```python
from build123d import *

# Parameters (mm, degrees)
CUT_EXTRUDE_1_DEPTH      = 192.109261942
CUT_EXTRUDE_1_DEPTH_BACK = 192.109261942
SKETCH_2_W               = 30
SKETCH_2_H               = 7.5
CHAMFER_1_SIZE           = 1.5
M8X1_01_D                = 7
M8X1_01_DEPTH            = 20
M8X1_01_CSINK_D          = 10
M8X1_01_CSINK_ANGLE      = 90
M8X1_01_TIP              = 2.103012167


with BuildPart() as part:
    # Эскиз1 → Повернуть1 (revolve)
    with BuildSketch(Plane.XY, mode=Mode.PRIVATE) as revolve_1_sk:
        Polygon((-186.5, 0), (-186.5, 25), (-82.5, 25), (-82.5, 29.5), (82.5, 29.5), (82.5, 25), (145.5, 25), (145.5, 0), align=None)
    revolve(revolve_1_sk.sketch.rotate(Axis((0, 0, 0), (-1, 0, 0)), 90), axis=Axis((0, 0, 0), (-1, 0, 0)))

    # Эскиз2 → Вырез-Вытянуть1 (cut, two sides: drawn at the far end of the back side and taken through both)
    with BuildSketch(Plane(origin=(0, 0, 0), x_dir=(1, 0, 0), z_dir=(0, 1, 0)).offset(-CUT_EXTRUDE_1_DEPTH_BACK)):
        with Locations((-171.5, 21.25)):
            Rectangle(SKETCH_2_W, SKETCH_2_H)
        with Locations((-171.5, -21.25)):
            Rectangle(SKETCH_2_W, SKETCH_2_H)
        with Locations((130.5, 21.25)):
            Rectangle(SKETCH_2_W, SKETCH_2_H)
        with Locations((130.5, -21.25)):
            Rectangle(SKETCH_2_W, SKETCH_2_H)
    extrude(amount=CUT_EXTRUDE_1_DEPTH + CUT_EXTRUDE_1_DEPTH_BACK, mode=Mode.SUBTRACT)

    # Фаска1
    chamfer_1_edges = [part.edges().sort_by_distance(p)[0] for p in [
        (145.5, 25, 0),
        (145.5, -25, 0),
        (-186.5, 25, 0),
        (-186.5, -25, 0),
        (82.5, 0, 29.5),
        (-82.5, 0, 29.5),
    ]]
    chamfer(chamfer_1_edges, length=CHAMFER_1_SIZE)

    # Отверстие обработанное метчиком M8x1.01
    with Locations(Plane(origin=(-172.5, 25, 0), x_dir=(0, 0, 1), z_dir=(0, 1, 0))):
        with Locations((0, 0), (0, 305)):
            CounterSinkHole(M8X1_01_D / 2, M8X1_01_CSINK_D / 2, depth=M8X1_01_DEPTH, counter_sink_angle=M8X1_01_CSINK_ANGLE)
            with Locations((0, 0, -(M8X1_01_DEPTH + M8X1_01_TIP / 2))):  # 118° drill point
                Cone(0, M8X1_01_D / 2, M8X1_01_TIP, mode=Mode.SUBTRACT)


solid = part.part
```
The model under review builds one solid part; all positions refer to its coordinate system, in mm. A direction names the side the tool comes from. Give positions to 0.01 mm unless a question says otherwise; leave off trailing zeros. Loops run counter-clockwise (first coordinate to the right, second up) from the corner with the lowest first, then second, coordinate; pieces in that order, holes last. Notation, with made-up numbers: (-5, 23.25) -> (-1, 23.25) arc R23 cw to (-1, 45.25) -> close; hole circle Ø1 at (5, -31). An arc over 180 degrees is marked (long way). Use CSV: the item, a comma, the result in double quotes.
1. To check wall thickness, follow probe 1 along X at (y, z) = (9, 0); probe 2 along Z at (x, y) = (132.5, 15); probe 3 along Y at (x, z) = (-78, -1). State the ranges of each line that lie inside material, in increasing order. Write a range as from..to.
Result:
probe 1,"x = -186.5..-176, -169..129, 136..145.5"
probe 2,"z = -17.5..-3.5, 3.5..17.5"
probe 3,"y = -29.48..29.48"
2. Consider section C-C, the plane x = -59.5. Write out the cut boundary in (y, z), then the cut area to 3 significant figures.
Result:
outline,"circle Ø59 at (0, 0)"
area,"2,730 mm²"
3. For P1, Ø2, axis at x = -96.5, y = -10.5, coming from the +Z side; P2, Ø2, axis at y = -6.5, z = 20.5, coming from the -X side; P3, Ø9, axis at x = 135, y = -5, coming from the -Z side, all flat-tipped, find the tip position at first contact; note any pin that passes through.
Result:
P1,"stops at z = 23.12"
P2,"stops at x = -156.5"
P3,"stops at z = -17.5"
4. Consider section B-B, the plane x = 124. Write out the cut boundary in (y, z), then the cut area to 3 significant figures.
Result:
outline,"(-17.85, -17.5) -> (17.85, -17.5) arc R25 ccw to (17.85, 17.5) -> (-17.85, 17.5) arc R25 ccw to start"
area,"1,590 mm²"
5. Machinability: for faces 1 (the face through (130, 0, 17.5)), 2 (the face through (-133.032, -7.509, -23.846)), 3 (the face through (-172, 0, 17.5)), 4 (the face through (130, 0, -17.5)), which of the approach directions +Z, -Z, +X, -X, +Y, -Y give a long, thin tool a straight path to every point of the face, cutting with its end or side? Answer none if there is none.
Result:
face 1,"+Z, +X, +Y, -Y"
face 2,"-X"
face 3,"+Z, -X, +Y, -Y"
face 4,"-Z, +X, +Y, -Y"
6. The part is to be moulded in two halves that separate along Z. For faces 5 (the face through (145.5, 0, 0)), 6 (the face through (-171.99, 3.26, 0.33)), 7 (the face through (-186, 24, 0)), say which applies: +Z half, -Z half, draft (parallel to the pull), parting line (faces both ways), or undercut.
Result:
face 5,"draft"
face 6,"undercut"
face 7,"parting line"
7. Consider section A-A, the plane y = 0. Write out the cut boundary in (x, z).
Result:
outline,"(-186.5, -17.5) -> (-156.5, -17.5) -> (-156.5, -25) -> (-82.5, -25) -> (-82.5, -28) -> (-81, -29.5) -> (81, -29.5) -> (82.5, -28) -> (82.5, -25) -> (115.5, -25) -> (115.5, -17.5) -> (145.5, -17.5) -> (145.5, 17.5) -> (115.5, 17.5) -> (115.5, 25) -> (82.5, 25) -> (82.5, 28) -> (81, 29.5) -> (-81, 29.5) -> (-82.5, 28) -> (-82.5, 25) -> (-156.5, 25) -> (-156.5, 17.5) -> (-186.5, 17.5) -> close"
